Autodesk Inventor part; units mm, degrees
ref_plane "YZ Plane" through (0, 0, 0) normal (1, 0, 0) x (0, 1, 0)
ref_plane "XZ Plane" through (0, 0, 0) normal (0, 1, 0) x (-1, 0, 0)
ref_plane "XY Plane" through (0, 0, 0) normal (0, 0, 1) x (1, 0, 0)
sketch "Sketch1" plane through (0, 0, 0) normal (0, 0, 1) x (1, 0, 0)
  circle A0 centre (0, 0) radius 22.5
  dimension "d0" = 45
extrude "Extrusion1" add sketch "Sketch1" along normal mid plane 19
sketch "Sketch2" plane through (0, 0, 9.5) normal (0, 0, 1) x (1, 0, 0)
  circle A0 centre (0, 0) radius 27.5
  circle A1 centre (0, 0) radius 22.5
  dimension "d3" = 5
extrude "Extrusion2" add sketch "Sketch2" against normal blind 2 contours A0 | A1
sketch "Sketch3" plane through (0, 0, -9.5) normal (0, 0, -1) x (-1, 0, 0)
  circle A0 centre (0, 0) radius 27.5
  circle A1 centre (0, 0) radius 22.5
extrude "Extrusion3" add sketch "Sketch3" against normal blind 2
sketch "Sketch4" plane through (0, 0, 9.5) normal (0, 0, 1) x (1, 0, 0)
  circle A0 centre (0, 0) radius 2.5
  line L0 (-1.5, 2) -> (1.5, 2)
  circle A1 centre (-1.5, 0.5) radius 1.5
  line L1 (0, 38.5) -> (0, -38.5)
  circle A2 centre (1.5, 0.5) radius 1.5
  point P0 (2.4, -0.7)
  point P1 (1.5, 2)
  point P2 (-2.4, -0.7)
  dimension "d25" = 3
  dimension "d8" = 5
  dimension "d9" = 4.5
extrude "Extrusion4" cut sketch "Sketch4" against normal through all contours A0 A2 | A0 A2 | A2 L1 L0 | A0 L1 A2 | L1 A1 L0 | A1 A0 | L1 A0 A1 | A0 A1
sketch "Sketch5" plane through (0, 0, -7.5) normal (0, 0, 1) x (1, 0, 0)
  line L0 (0, -38.5) -> (0, 38.5)
  circle A0 centre (0, 24) radius 1.5
  circle A1 centre (0, 0) radius 22.5
  dimension "d31" = 3
extrude "Extrusion5" cut sketch "Sketch5" against normal through all contours A0 L0 | L0 A0
pattern_circular "Circular Pattern1" count 12 over 360 about axis through (0, 0, -10) along (0, 0, 1) of "Extrusion5"
properties part number "WinderSpoolTraditionalMachining"
Model file for the job. Use its own axes, mm. A direction names the side the tool comes from. Give positions to 0.01 mm unless a question says otherwise; leave off trailing zeros. Loops run counter-clockwise (first coordinate to the right, second up) from the corner with the lowest first, then second, coordinate; pieces in that order, holes last. Notation, with made-up numbers: (-11.75, 16.25) - (1.25, 16.25) arc R21 ccw to (1.25, 36.25) - close; hole circle Ø5 at (-38.75, 21). An arc over 180 degrees is marked (long way). One line per item, written item: value. Start each with the question number.
1. Pull direction Z, two halves, no side cores. Call faces 4 (the flat face through (-23, 0, 7.5)), 5 (the cylindrical face through (19.59, -12.91, -8.49)), 6 (the flat face through (0, -6, -9.5)), 7 (the flat face through (4.2, -22.3, -7.5)): pulls with the +Z half, pulls with the -Z half, needs draft (parallel to the pull), parting line crosses it, or undercut.
2. Slice it at A-A (y = 24). List the corners of the cut face in (x, z).
3. Pin check, flat tips, straight feed: pin 1 (1 mm diameter, centred on x = -0.5, z = 5.5, fed in from +Y); pin 2 (1.5 mm diameter, centred on x = 0.5, z = -1, fed in from -Y); pin 3 (1.8 mm diameter, centred on x = 20.78, y = -12, fed in from -Z). Stop position of each tip, or through.
4. Probe L1, parallel to X at y = -12, z = -8.05; L2, parallel to Y at x = 19.5, z = -8; L3, parallel to Y at x = 22, z = -8.5. List the from-to ranges inside material, lowest first. Write a range as from..to.
5. Slice it at B-B (z = -5). List the corners of the cut face in (x, y).
6. Which spindle directions (+Z, -Z, +X, -X, +Y, -Y) get a long thin tool onto all of the face, cutting with end or side? Do faces 1 (the cylindrical face through (0, -2.5, 0.1)), 2 (the cylindrical face through (10.382, 19.961, -0.105)), 3 (the cylindrical face through (-19.59, 12.91, -8.49)). Say none if no direction does.
7. Slice it at D-D (x = 6). List the corners of the cut face in (y, z), plus the area to 3 significant figures.
Solution:
1. face 4: undercut
1. face 5: needs draft
1. face 6: pulls with the -Z half
1. face 7: undercut
2. outline: (-13.43, -9.5) - (-1.5, -9.5) - (-1.5, -7.5) - (-13.43, -7.5) - close; (-13.43, 7.5) - (13.43, 7.5) - (13.43, 9.5) - (-13.43, 9.5) - close; (1.5, -9.5) - (13.43, -9.5) - (13.43, -7.5) - (1.5, -7.5) - close
3. pin 1: stops at y = 22.5
3. pin 2: stops at y = -22.5
3. pin 3: stops at z = 7.5
4. L1: x = -24.74..-22.28, -19.28..19.28, 22.28..24.74
4. L2: y = -19.39..-12.77, -11.23..11.23, 12.77..19.39
4. L3: y = -16.5..-12.88, -11.12..11.12, 12.88..16.5
5. outline: circle Ø45 at (0, 0); hole (-2.4, -0.7) arc R2.5 ccw to (2.4, -0.7) arc R1.5 ccw to (1.5, 2) - (-1.5, 2) arc R1.5 ccw to start
6. face 1: +Z, -Z
6. face 2: none
6. face 3: -Z
7. outline: (-26.84, -9.5) - (26.84, -9.5) - (26.84, -7.5) - (21.69, -7.5) - (21.69, 7.5) - (26.84, 7.5) - (26.84, 9.5) - (-26.84, 9.5) - (-26.84, 7.5) - (-21.69, 7.5) - (-21.69, -7.5) - (-26.84, -7.5) - close
7. area: 865 mm^2
